```python
from build123d import *

# Parameters (mm, degrees)
Y_KSEKLIK_EKSTR_ZYON1_DEPTH = 10


# Read off the part's stored shape, not the designer's step: Döndür-İnce1
with BuildPart() as part:
    # Döndür-İnce1 outline → Döndür-İnce1 (revolve)
    with BuildSketch(Plane.XZ):
        with BuildLine():
            Line((0, 265.5), (0, 255.5))
            Line((0, 255.5), (45, 255.5))
            Line((45, 255.5), (45, 67.5))
            Line((45, 67.5), (120, 67.5))
            Line((120, 67.5), (120, -67.5))
            Line((120, -67.5), (107.149606299, -67.5))
            Line((107.149606299, -67.5), (107.149606299, 7.5))
            Line((107.149606299, 7.5), (87.149606299, 7.5))
            Line((87.149606299, 7.5), (87.149606299, -32.5))
            ThreePointArc((87.149606299, -32.5), (81.291741923, -46.642135624), (67.149606299, -52.5))
            Line((67.149606299, -52.5), (57.149606299, -52.5))
            ThreePointArc((57.149606299, -52.5), (43.007470675, -46.642135624), (37.149606299, -32.5))
            Line((37.149606299, -32.5), (37.149606299, 7.5))
            Line((37.149606299, 7.5), (17.149606299, 7.5))
            Line((17.149606299, 7.5), (17.149606299, -67.5))
            Line((17.149606299, -67.5), (0, -67.5))
            Line((0, -67.5), (0, -77.5))
            Line((0, -77.5), (27.149606299, -77.5))
            Line((27.149606299, -77.5), (27.149606299, -32.5))
            ThreePointArc((27.149606299, -32.5), (35.936402864, -53.713203435), (57.149606299, -62.5))
            Line((57.149606299, -62.5), (67.149606299, -62.5))
            ThreePointArc((67.149606299, -62.5), (88.362809735, -53.713203436), (97.149606299, -32.5))
            Line((97.149606299, -32.5), (97.149606299, -77.5))
            Line((97.149606299, -77.5), (130, -77.5))
            Line((130, -77.5), (130, 77.5))
            Line((130, 77.5), (55, 77.5))
            Line((55, 77.5), (55, 265.5))
            Line((55, 265.5), (0, 265.5))
        make_face()
    revolve(axis=Axis((0, 0, 0), (0, 0, 1)))

    # Çizim2 → Yükseklik-Ekstrüzyon1 (add)
    with BuildSketch(Plane(origin=(0, 0, -62.5), x_dir=(-1, 0, 0), z_dir=(0, 0, -1))):
        Polygon((62.149606299, -13.529902504), (71.716692108, -9.567085809), (75.679508803, 0), (71.716692108, 9.567085809), (62.149606299, 13.529902504), (52.58252049, 9.567085809), (48.619703796, 0), (52.58252049, -9.567085809), align=None)
        Polygon((53.513493871, -53.513493871), (57.476310566, -43.946408062), (53.513493871, -34.379322253), (43.946408062, -30.416505559), (34.379322253, -34.379322253), (30.416505559, -43.946408062), (34.379322253, -53.513493871), (43.946408062, -57.476310566), align=None)
        Polygon((0, -75.679508803), (9.567085809, -71.716692108), (13.529902504, -62.149606299), (9.567085809, -52.58252049), (0, -48.619703796), (-9.567085809, -52.58252049), (-13.529902504, -62.149606299), (-9.567085809, -71.716692108), align=None)
        Polygon((-53.513493871, -53.513493871), (-43.946408062, -57.476310566), (-34.379322253, -53.513493871), (-30.416505559, -43.946408062), (-34.379322253, -34.379322253), (-43.946408062, -30.416505559), (-53.513493871, -34.379322253), (-57.476310566, -43.946408062), align=None)
        Polygon((-75.679508803, 0), (-71.716692108, -9.567085809), (-62.149606299, -13.529902504), (-52.58252049, -9.567085809), (-48.619703796, 0), (-52.58252049, 9.567085809), (-62.149606299, 13.529902504), (-71.716692108, 9.567085809), align=None)
        Polygon((-53.513493871, 53.513493871), (-57.476310566, 43.946408062), (-53.513493871, 34.379322253), (-43.946408062, 30.416505559), (-34.379322253, 34.379322253), (-30.416505559, 43.946408062), (-34.379322253, 53.513493871), (-43.946408062, 57.476310566), align=None)
        Polygon((0, 75.679508803), (-9.567085809, 71.716692108), (-13.529902504, 62.149606299), (-9.567085809, 52.58252049), (0, 48.619703796), (9.567085809, 52.58252049), (13.529902504, 62.149606299), (9.567085809, 71.716692108), align=None)
        Polygon((53.513493871, 53.513493871), (43.946408062, 57.476310566), (34.379322253, 53.513493871), (30.416505559, 43.946408062), (34.379322253, 34.379322253), (43.946408062, 30.416505559), (53.513493871, 34.379322253), (57.476310566, 43.946408062), align=None)
    extrude(amount=Y_KSEKLIK_EKSTR_ZYON1_DEPTH)


solid = part.part
```
Could you check a few things on this model? Use its own coordinates, in mm. A direction names the side the tool comes from. Round coordinates to 2 decimals unless told otherwise and drop trailing zeros. Loops run counter-clockwise (first coordinate to the right, second up) from the corner with the lowest first, then second, coordinate; pieces in that order, holes last. Notation, with made-up numbers: M -18.5,-17 L 21.5,-17 A32 cw 21.5,15 Z; hole C 71,-31 d11. An arc over 180 degrees is marked long. Write item = value, one per line.
1. I want a section at B-B, the plane z = 50. Write out the boundary of the cut face in (x, y).
Results below:
outline = C 0,0 d260; hole C 0,0 d240
2. I need wall thicknesses on probe 1 along Y at (x, z) = (0, -12); probe 2 along Z at (x, y) = (0, 105); probe 3 along Y at (x, z) = (0, 214.5). Which ranges of each line are inside material? Lowest first, please.
Results below:
probe_1 = -130 to -120, -107.15 to -87.15, -37.15 to -17.15, 17.15 to 37.15, 87.15 to 107.15, 120 to 130
probe_2 = -77.5 to 7.5, 67.5 to 77.5
probe_3 = -55 to -45, 45 to 55
3. Which directions (+Z, -Z, +X, -X, +Y, -Y) give clear straight access to the entire face, cutting with the end or side of a thin tool? Please do faces 1 (the face through (35.434, 11.159, -12.22)), 2 (the face through (39.096, -32.426, -67.43)).
Results below:
face_1 = none
face_2 = -Z
4. Will these pins go through, and if not, where does the flat tip stop? P1, Ø8, axis at x = -45.5, y = 49, coming from the -Z side; P2, Ø7.5, axis at x = -72, y = -5.5, coming from the +Z side; P3, Ø4, axis at x = 43.5, y = 3, coming from the -Z side.
Results below:
P1 = -72.5
P2 = 77.5
P3 = -60.19
5. I want a section at A-A, the plane z = 117. Write out the boundary of the cut face in (x, y), and give its area (3 significant figures).
Results below:
outline = C 0,0 d110; hole C 0,0 d90
area = 3,140 mm²
